from build123d import *

# Parameters (mm, degrees)
F0_W     = 3.175
F0_H     = 8.89
F0_H_2   = 12.7
F0_H_3   = 49.53
F0_H_4   = 27.94
F0_W_2   = 8.89
F0_H_5   = 11.43
F0_W_3   = 12.7
F0_H_6   = 3.175
F1_DEPTH = 3.175


with BuildPart() as f1:
    # F0 (on Front) → F1 (new body)
    with BuildSketch(Plane.XZ):
        with BuildLine():
            Line((-38.175, 76.2), (-47.625, 76.2))
            Line((-47.625, 76.2), (-47.625, 67.31))
            Line((-47.625, 67.31), (-47.625, 58.42))
            Line((-47.625, 58.42), (-47.625, 49.53))
            Line((-47.625, 49.53), (-47.625, 40.64))
            Line((-47.625, 40.64), (-47.625, 27.94))
            Line((-47.625, 27.94), (-47.625, 0))
            Line((-47.625, 0), (-50.8, 0))
            Line((-50.8, 0), (-50.8, -50.8))
            Line((-50.8, -50.8), (-43.18, -50.8))
            Line((-43.18, -50.8), (-43.18, -41.91))
            Line((-43.18, -41.91), (-34.29, -41.91))
            Line((-34.29, -41.91), (-34.29, -50.8))
            Line((-34.29, -50.8), (-31.75, -50.8))
            ThreePointArc((-31.75, -50.8), (0, -19.05), (31.75, -50.8))
            Line((31.75, -50.8), (50.8, -50.8))
            Line((50.8, -50.8), (50.8, 0))
            Line((50.8, 0), (47.625, 0))
            Line((47.625, 0), (47.625, 12.7))
            Line((47.625, 12.7), (47.625, 25.4))
            Line((47.625, 25.4), (47.625, 38.1))
            Line((47.625, 38.1), (47.625, 49.53))
            Line((47.625, 49.53), (47.625, 58.42))
            Line((47.625, 58.42), (47.625, 67.31))
            Line((47.625, 67.31), (47.625, 76.2))
            Line((47.625, 76.2), (38.175, 76.2))
            Line((38.175, 76.2), (38.175, 67.31))
            Line((38.175, 67.31), (38.175, 58.42))
            Line((38.175, 58.42), (38.175, 49.53))
            Line((38.175, 49.53), (38.175, 40.64))
            Line((38.175, 40.64), (38.175, 27.94))
            Line((38.175, 27.94), (38.175, 0))
            Line((38.175, 0), (35, 0))
            Line((35, 0), (35, 27.94))
            Line((35, 27.94), (35, 40.64))
            Line((35, 40.64), (35, 49.53))
            Line((35, 49.53), (35, 58.42))
            Line((35, 58.42), (35, 67.31))
            Line((35, 67.31), (35, 76.2))
            Line((35, 76.2), (-35, 76.2))
            Line((-35, 76.2), (-35, 67.31))
            Line((-35, 67.31), (-35, 58.42))
            Line((-35, 58.42), (-35, 49.53))
            Line((-35, 49.53), (-35, 0))
            Line((-35, 0), (-38.175, 0))
            Line((-38.175, 0), (-38.175, 49.53))
            Line((-38.175, 49.53), (-38.175, 58.42))
            Line((-38.175, 58.42), (-38.175, 67.31))
            Line((-38.175, 67.31), (-38.175, 76.2))
        make_face()
        Polygon((19.05, -1.975), (31.75, -1.975), (31.75, -5.15), (19.05, -5.15), (6.35, -5.15), (-6.35, -5.15), (-19.05, -5.15), (-31.75, -5.15), (-31.75, -1.975), (-19.05, -1.975), (-6.35, -1.975), (6.35, -1.975), align=None, mode=Mode.SUBTRACT)
        Polygon((19.05, 21.2), (31.75, 21.2), (31.75, 18.025), (19.05, 18.025), (6.35, 18.025), (-6.35, 18.025), (-19.05, 18.025), (-31.75, 18.025), (-31.75, 21.2), (-19.05, 21.2), (-6.35, 21.2), (6.35, 21.2), align=None, mode=Mode.SUBTRACT)
        with Locations((-49.2125, 62.865)):
            Rectangle(F0_W, F0_H)
        with Locations((-36.5875, 62.865)):
            Rectangle(F0_W, F0_H)
        with Locations((-49.2125, 45.085)):
            Rectangle(F0_W, F0_H)
        with Locations((-49.2125, 34.29)):
            Rectangle(F0_W, F0_H_2)
        with Locations((36.5875, 62.865)):
            Rectangle(F0_W, F0_H)
        with Locations((-36.5875, 24.765)):
            Rectangle(F0_W, F0_H_3)
        with Locations((-49.2125, 13.97)):
            Rectangle(F0_W, F0_H_4)
        with Locations((49.2125, 62.865)):
            Rectangle(F0_W, F0_H)
        with Locations((36.5875, 45.085)):
            Rectangle(F0_W, F0_H)
        with Locations((36.5875, 34.29)):
            Rectangle(F0_W, F0_H_2)
        with Locations((-38.735, -46.355)):
            Rectangle(F0_W_2, F0_H)
        with Locations((49.2125, 43.815)):
            Rectangle(F0_W, F0_H_5)
        with Locations((36.5875, 13.97)):
            Rectangle(F0_W, F0_H_4)
        with Locations((49.2125, 31.75)):
            Rectangle(F0_W, F0_H_2)
        with Locations((49.2125, 19.05)):
            Rectangle(F0_W, F0_H_2)
        with Locations((49.2125, 6.35)):
            Rectangle(F0_W, F0_H_2)
        with Locations((25.4, 19.6125)):
            Rectangle(F0_W_3, F0_H_6)
        with Locations((12.7, 19.6125)):
            Rectangle(F0_W_3, F0_H_6)
        with Locations((-12.7, 19.6125)):
            Rectangle(F0_W_3, F0_H_6)
        with Locations((-25.4, 19.6125)):
            Rectangle(F0_W_3, F0_H_6)
        with Locations((25.4, -3.5625)):
            Rectangle(F0_W_3, F0_H_6)
        with Locations((12.7, -3.5625)):
            Rectangle(F0_W_3, F0_H_6)
        with Locations((-12.7, -3.5625)):
            Rectangle(F0_W_3, F0_H_6)
        with Locations((-25.4, -3.5625)):
            Rectangle(F0_W_3, F0_H_6)
    extrude(amount=F1_DEPTH)


solid = f1.part
Geometry check sheet. Reference: the model listing, model coordinates, mm. A direction names the side the tool comes from. Coordinates: 2 decimals unless noted, no trailing zeros. Order: outer loops, then holes, each group sorted by start corner. A loop starts at its lowest first (then second) coordinate and runs counter-clockwise, first axis right, second up. Notation, with made-up numbers: (-40, 18) - (-19, 18) arc R19 ccw to (-19, 49) - close; hole circle Ø7 at (78.5, 2). An arc over 180 degrees is marked (long way). One line per item, written item: value.
(1) Access from +Z, -Z, +X, -X, +Y, -Y to the whole of each face (thin tool, end or side, straight path). Record for faces 5 (the face through (0, -2, 21.2)), 6 (the face through (-47.625, -2, 72)), 7 (the face through (49, -2, 67.31)), 8 (the face through (-49, -2, 58.42)), 9 (the face through (49, -2, 49.53)).
Data:
face 5: +Y, -Y
face 6: +Z, -X, +Y, -Y
face 7: +Z, +X, +Y, -Y
face 8: -X, +Y, -Y
face 9: +X, +Y, -Y
(2) Sectioned sample at A-A (z = 52.5). Enter the section's corners in (x, y) (3 decimals).
Data:
outline: (-47.625, -3.175) - (-38.175, -3.175) - (-38.175, 0) - (-47.625, 0) - close; (-35, -3.175) - (35, -3.175) - (35, 0) - (-35, 0) - close; (38.175, -3.175) - (47.625, -3.175) - (47.625, 0) - (38.175, 0) - close
(3) Sectioned sample at B-B (x = 0). Enter the section's corners in (y, z) (3 decimals), and give its area (3 significant figures).
Data:
outline: (-3.175, -19.05) - (0, -19.05) - (0, -5.15) - (-3.175, -5.15) - close; (-3.175, -1.975) - (0, -1.975) - (0, 18.025) - (-3.175, 18.025) - close; (-3.175, 21.2) - (0, 21.2) - (0, 76.2) - (-3.175, 76.2) - close
area: 282 mm^2
(4) Depth check by flat-ended pin: pin 1 Ø1.6 at (y, z) = (-1.5, 56) entering from +X (3 decimals); pin 2 Ø1.6 at (y, z) = (-1, 53) entering from -X (3 decimals); pin 3 Ø1.5 at (x, y) = (14, -0.5) entering from -Z. Enter the tip coordinate at first touch or a pass-through.
Data:
pin 1: stops at x = 47.625
pin 2: stops at x = -47.625
pin 3: stops at z = -22.68
(5) Sectioned sample at C-C (z = -31). Enter the section's corners in (x, y) (3 decimals), and give its area (3 significant figures).
Data:
outline: (-50.8, -3.175) - (-24.82, -3.175) - (-24.82, 0) - (-50.8, 0) - close; (24.82, -3.175) - (50.8, -3.175) - (50.8, 0) - (24.82, 0) - close
area: 165 mm^2
(6) Thickness scan on probe 1 along X at (y, z) = (-1.75, 68.5) (3 decimals); probe 2 along Z at (x, y) = (0, -2.9) (3 decimals); probe 3 along Z at (x, y) = (-36, -2.3). Record the ranges inside material, lowest first. Write a range as from..to.
Data:
probe 1: x = -47.625..-38.175, -35..35, 38.175..47.625
probe 2: z = -19.05..-5.15, -1.975..18.025, 21.2..76.2
probe 3: z = -50.8..49.53, 58.42..67.31
(7) Release check for a two-part mould opening along Z. For faces 1 (the face through (-49, -2, 67.31)), 2 (the face through (-1, 0, 14)), 3 (the face through (6.35, -2, -4)), 4 (the face through (0, -2, 18.025)) record: +Z half, -Z half, draft (parallel to the pull), parting line (faces both ways), or undercut.
Data:
face 1: +Z half
face 2: draft
face 3: undercut
face 4: undercut
(8) Sectioned sample at D-D (y = -0.95). Count the separate pieces of the cut face and the enclosed holes in it, and give its area (3 significant figures).
Data:
separate pieces: 1
enclosed holes: 4
area: 11,000 mm^2
